Can you work these out from the model? Positions are in its coordinate system, mm. A direction names the side the tool comes from. Give positions to 0.01 mm unless a question says otherwise; leave off trailing zeros. Loops run counter-clockwise (first coordinate to the right, second up) from the corner with the lowest first, then second, coordinate; pieces in that order, holes last. Notation, with made-up numbers: (-36, -30) - (14, -30) arc R25 ccw to (14, -16) - close; hole circle Ø10 at (-11.5, 37). An arc over 180 degrees is marked (long way). Use a Markdown table: item, result. Add a question column.
Autodesk Inventor part; units mm, degrees
ref_plane "YZ Plane" through (0, 0, 0) normal (1, 0, 0) x (0, 1, 0)
ref_plane "XZ Plane" through (0, 0, 0) normal (0, 1, 0) x (-1, 0, 0)
ref_plane "XY Plane" through (0, 0, 0) normal (0, 0, 1) x (1, 0, 0)
sketch "Sketch1" plane through (0, 0, 0) normal (0, 1, 0) x (-1, 0, 0)
  circle A0 centre (69.3, 81.8) radius 2.75
  circle A1 centre (69.3, -81.8) radius 2.75
  circle A2 centre (-69.3, -81.8) radius 2.75
  circle A3 centre (-69.3, 81.8) radius 2.75
  line L0 (69.3, 81.8) -> (-69.3, 81.8) construction
  line L1 (69.3, 81.8) -> (69.3, -81.8) construction
  line L2 (69.3, -81.8) -> (-69.3, -81.8) construction
  line L3 (0, 0) -> (69.3, 0) construction
  line L4 (-83, -133) -> (83, -133)
  line L5 (83, -133) -> (83, 133)
  line L6 (83, 133) -> (-83, 133)
  line L7 (-83, 133) -> (-83, -133)
  line L8 (-83, -133) -> (83, 133) construction
  line L9 (83, -133) -> (-83, 133) construction
  circle A4 centre (75, 125) radius 2.75
  circle A5 centre (-75, 125) radius 2.75
  circle A6 centre (-75, -125) radius 2.75
  circle A7 centre (75, -125) radius 2.75
  line L10 (75, 125) -> (-75, 125) construction
  line L11 (-75, 125) -> (-75, -125) construction
  line L12 (75, -125) -> (-75, -125) construction
  circle A8 centre (69.3, 81.8) radius 5
  circle A9 centre (-69.3, 81.8) radius 5
  circle A10 centre (-69.3, -81.8) radius 5
  circle A11 centre (69.3, -81.8) radius 5
  point P0 (0, 81.8)
  dimension "d0" = 163.6
  dimension "d1" = 5.5
  dimension "d2" = 138.6
  dimension "d3" = 69.3
  dimension "d4" = 5.5
  dimension "d5" = 10
  dimension "d7" = 250
  dimension "d8" = 8
  dimension "d9" = 8
  dimension "d10" = 8
  dimension "d11" = 8
  dimension "d12" = 8
  dimension "d13" = 150
extrude "Extrusion1" add sketch "Sketch1" along normal blind 10 contours L7 L6 L5 L4
extrude "Extrusion2" add sketch "Sketch1" along normal blind 3 contours A8 | A9 | A10 | A11
sketch "Sketch2" plane through (0, 10, 0) normal (0, 1, 0) x (1, 0, 0)
  line L0 (-83, 133) -> (-83, -133)
  line L1 (-83, -133) -> (83, -133)
  line L2 (83, -133) -> (83, 133)
  line L3 (83, 133) -> (-83, 133)
  circle A0 centre (-75, -125) radius 2.75
  circle A1 centre (75, -125) radius 2.75
  circle A2 centre (75, 125) radius 2.75
  circle A3 centre (-75, 125) radius 2.75
  circle A4 centre (-69.3, 81.8) radius 5
  circle A5 centre (69.3, 81.8) radius 5
  circle A6 centre (69.3, -81.8) radius 5
  circle A7 centre (-69.3, -81.8) radius 5
  arc A8 (60, -133) -> (-60, -133) centre (0, -133) ccw
  line L4 (0, -73) -> (0, -133) construction
  arc A9 (83, 70) -> (83, -70) centre (83, 0) ccw
  line L5 (13, 0) -> (83, 0) construction
  line L6 (83, -133) -> (83, 133) construction
  arc A10 (-83, -70) -> (-83, 70) centre (-83, 0) ccw
  arc A11 (-60, 133) -> (60, 133) centre (0, 133) ccw
  point P0 (0, 0)
  point P1 (-60, 133)
  point P2 (60, 133)
  point P3 (-83, 70)
  dimension "d18" = 70
  dimension "d19" = 60
extrude "Extrusion3" cut sketch "Sketch2" against normal through all contours A10 L0 | L3 A11 | A8 L1 | L2 A9
fillet "Fillet1" radius 10 12 edges at (60, 5, 133) (-60, 5, 133) (83, 5, 133) (83, 5, -70) (83, 5, 70) (-83, 5, 133) (-83, 5, 70) (-83, 5, -70) (-83, 5, -133) (60, 5, -133) (-60, 5, -133) (83, 5, -133)
equation "\"d3\" = 0.5 * d2"
equation "\"d9\" = d8"
equation "\"d10\" = d9"
equation "\"d11\" = d8"
equation "\"d12\" = d8"
properties part number "Spincoater Base Mount_3DPrint"
1. If we mould it in two halves opening along X, with no side actions, what happens to faces 1 (the face through (-70.78, 1.48, 79.48)), 2 (the face through (-6, 0, 1)), 3 (the face through (-83, 5, -101))? For each: released by +X, released by -X, zero draft, split by the parting line, or undercut.
2. Suppose I cut it at A-A (y = 5.75). State how many separate pieces and enclosed holes the cut face has, and give its area (3 significant figures).
3. Suppose I cut it at D-D (x = 0). List the corners of the cut face in (y, z) for me.
4. Will these pins go through, and if not, where does the flat tip stop? P1, Ø8, axis at x = 69.5, z = -81, coming from the +Y side; P2, Ø1, axis at x = -26, y = 6.5, coming from the -Z side; P3, Ø6, axis at x = -28.5, y = 7, coming from the -Z side.
5. Suppose I cut it at B-B (x = -25). List the corners of the cut face in (y, z) for me.
6. Suppose I cut it at C-C (x = -42). List the corners of the cut face in (y, z) for me.
7. Please list where these lines run through material, in increasing order: line 1 along Z through (x, y) = (69.3, 4.5); line 2 along Z through (x, y) = (-75, 7); line 3 along X through (y, z) = (7.75, 84). Write a range as [from, to].
8. On a 3-axis mill with a long thin cutter (end or side, diameter ignored), from which of +Z, -Z, +X, -X, +Y, -Y can I reach the whole of each face in a straight line? I mean faces 4 (the face through (62.811, 4.93, 130.624)), 5 (the face through (79.99, 5.07, 130.15)), 6 (the face through (-62.811, 4.93, -130.624)), 7 (the face through (80.567, 4.93, -72.834)), 8 (the face through (-71.988, 6.451, -86.016)). Say none if no direction works.
Results below:
| question | item | result |
|---|---|---|
| 1 | face 1 | undercut |
| 1 | face 2 | zero draft |
| 1 | face 3 | released by -X |
| 2 | separate pieces | 1 |
| 2 | enclosed holes | 8 |
| 2 | area | 16,800 mm² |
| 3 | outline | (0, -73) - (10, -73) - (10, 73) - (0, 73) - close |
| 4 | P1 | y = 3 |
| 4 | P2 | z = -79.17 |
| 4 | P3 | z = -81.93 |
| 5 | outline | (0, -78.46) - (10, -78.46) - (10, -39.19) - (0, -39.19) - close; (0, 39.19) - (10, 39.19) - (10, 78.46) - (0, 78.46) - close |
| 6 | outline | (0, -90.15) - (10, -90.15) - (10, -56.74) - (0, -56.74) - close; (0, 56.74) - (10, 56.74) - (10, 90.15) - (0, 90.15) - close |
| 7 | line 1 | [-133, -86.8], [-76.8, -68.65], [68.65, 76.8], [86.8, 133] |
| 7 | line 2 | [-132.8, -127.75], [-122.25, -69.57], [69.57, 122.25], [127.75, 132.8] |
| 7 | line 3 | [-83, -73.79], [-64.81, -34.63], [34.63, 64.81], [73.79, 83] |
| 8 | face 4 | +Z, +Y, -Y |
| 8 | face 5 | +Z, +X, +Y, -Y |
| 8 | face 6 | -Z, +Y, -Y |
| 8 | face 7 | +X, +Y, -Y |
| 8 | face 8 | +Y |
